from build123d import *

# Parameters (mm, degrees)
ESQUISSE1_W             = 20
ESQUISSE1_H             = 40
ESQUISSE1_R             = 2.75
BOSS_EXTRU_1_DEPTH      = 5
BOSS_EXTRU_2_DEPTH      = 10
ENL_V_MAT_EXTRU_1_REACH = 46.697
ESQUISSE3_R             = 1


with BuildPart() as part:
    # Esquisse1 → Boss.-Extru.1 (new body)
    with BuildSketch(Plane.XY):
        with Locations((-27.825146679, -3.282272289)):
            Rectangle(ESQUISSE1_W, ESQUISSE1_H)
        with Locations((-27.825146679, 6.717727711)):
            Circle(ESQUISSE1_R, mode=Mode.SUBTRACT)
        with Locations((-27.825146679, -13.282272289)):
            Circle(ESQUISSE1_R, mode=Mode.SUBTRACT)
    extrude(amount=BOSS_EXTRU_1_DEPTH)

    # Esquisse2 → Boss.-Extru.2 (add)
    with BuildSketch(Plane.XZ.offset(23.282272289)):
        Polygon((-17.825146679, 0), (-17.825146679, 5), (-12.825146679, 0), (9.063128198, 0), (9.063128198, -5), (-12.825146679, -5), align=None)
    extrude(amount=-BOSS_EXTRU_2_DEPTH)

    # Esquisse3 → Enlèv. mat.-Extru.1 (cut, up to next)
    with BuildSketch(Plane.XY, mode=Mode.PRIVATE) as enl_v_mat_extru_1_sk1:
        with Locations((4.063128198, -18.282272289)):
            Circle(ESQUISSE3_R)
    enl_v_mat_extru_1_tool1 = extrude(enl_v_mat_extru_1_sk1.sketch, amount=-ENL_V_MAT_EXTRU_1_REACH, mode=Mode.PRIVATE) & part.part
    # Esquisse3 → Enlèv. mat.-Extru.1 (cut, up to next)
    with BuildSketch(Plane.XY, mode=Mode.PRIVATE) as enl_v_mat_extru_1_sk2:
        with Locations((-5.436871802, -18.282272289)):
            Circle(ESQUISSE3_R)
    enl_v_mat_extru_1_tool2 = extrude(enl_v_mat_extru_1_sk2.sketch, amount=-ENL_V_MAT_EXTRU_1_REACH, mode=Mode.PRIVATE) & part.part
    add(enl_v_mat_extru_1_tool1.solids().sort_by_distance((4.063128, -18.282272, 0))[0], mode=Mode.SUBTRACT)
    add(enl_v_mat_extru_1_tool2.solids().sort_by_distance((-5.436872, -18.282272, 0))[0], mode=Mode.SUBTRACT)


solid = part.part
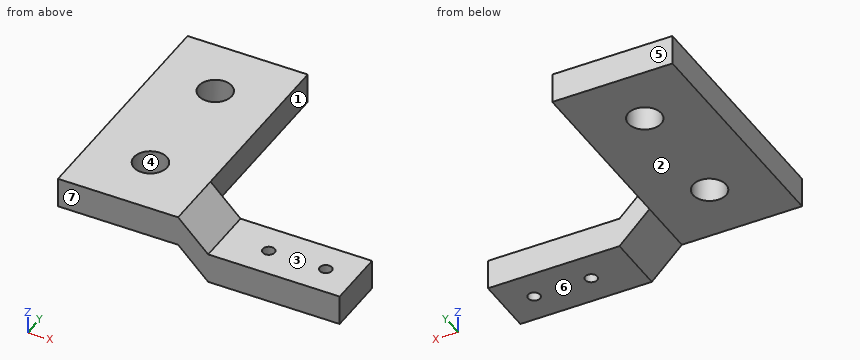
Verification items for the finished model (mm, model axes). Face numbers are marked on the shaded views. A direction names the side the tool comes from. Coordinates: 2 decimals unless noted, no trailing zeros. Order: outer loops, then holes, each group sorted by start corner. A loop starts at its lowest first (then second) coordinate and runs counter-clockwise, first axis right, second up. Notation, with made-up numbers: M 57,-21 L 64,-21 A17 ccw 64,-15 Z; hole C 74.5,28 d2. An arc over 180 degrees is marked long. One line per item, written item: value. Start each with the question number.
Item 1: Sectioned sample at B-B (y = 6). Enter the section's corners in (x, z), then the cut area to 3 significant figures.
Item 2: Access from +Z, -Z, +X, -X, +Y, -Y to the whole of each face (thin tool, end or side, straight path). Record for the marked faces 1, 2 and 3.
Item 3: Sectioned sample at A-A (x = -27). Enter the section's corners in (y, z).
Item 4: Sectioned sample at C-C (z = 2.5). Enter the section's corners in (x, y).
Item 5: Mould release check, pull along Y, two halves, no side actions. Record for the marked faces 4, 5, 6 and 7: released by +Y, released by -Y, zero draft, split by the parting line, or undercut.
Item 6: Sectioned sample at D-D (x = -5). Enter the section's corners in (y, z).
Item 7: Gauge pin test, flat ends, axial feed: pin 1 (3 mm diameter, centred on x = -5, z = -1, fed in from +Y); pin 2 (1.5 mm diameter, centred on y = -5, z = 2.5, fed in from +X); pin 3 (8 mm diameter, centred on x = -3.5, y = -20.5, fed in from +Z). Record the tip position at first contact, or that the pin passes through.
Item 8: Scan lines: probe 1 along Y at (x, z) = (-30, 3); probe 2 along Y at (x, z) = (4, -2.25); probe 3 along Z at (x, y) = (-0.5, -16.5). Record each from-to range of solid material in increasing order.
Conclusion:
1. outline: M -37.83,0 L -30.48,0 L -30.48,5 L -37.83,5 Z; M -25.17,0 L -17.83,0 L -17.83,5 L -25.17,5 Z
1. area: 73.5 mm^2
2. face 1: +Z, -Z, +X, +Y
2. face 2: -Z, -X, +Y, -Y
2. face 3: +Z, +X, +Y, -Y
3. outline: M -23.28,0 L -15.91,0 L -15.91,5 L -23.28,5 Z; M -10.66,0 L 4.09,0 L 4.09,5 L -10.66,5 Z; M 9.34,0 L 16.72,0 L 16.72,5 L 9.34,5 Z
4. outline: M -37.83,-23.28 L -15.33,-23.28 L -15.33,-13.28 L -17.83,-13.28 L -17.83,16.72 L -37.83,16.72 Z; hole C -27.83,-13.28 d5.5; hole C -27.83,6.72 d5.5
5. face 4: undercut
5. face 5: released by +Y
5. face 6: zero draft
5. face 7: released by -Y
6. outline: M -23.28,-5 L -19.18,-5 L -19.18,0 L -23.28,0 Z; M -17.38,-5 L -13.28,-5 L -13.28,0 L -17.38,0 Z
7. pin 1: stops at y = -13.28
7. pin 2: stops at x = -17.83
7. pin 3: stops at z = 0
8. probe 1: y = -23.28 to -14.97, -11.6 to 5.03, 8.4 to 16.72
8. probe 2: y = -23.28 to -19.28, -17.28 to -13.28
8. probe 3: z = -5 to 0
